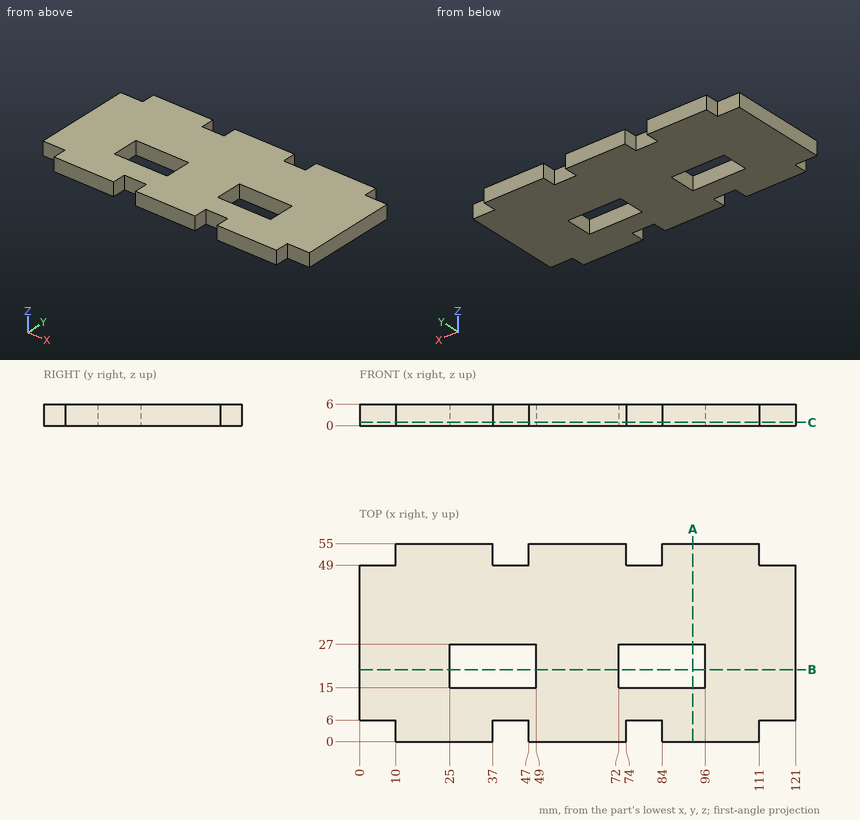
The drawing under review shows one solid part. Ordinate dimensions are in mm from its lowest x, y, z. Round coordinates to 2 decimals unless told otherwise and drop trailing zeros. Write each loop counter-clockwise with the first axis right and the second up, starting at its lowest first coordinate (ties: lowest second). Pieces come first, ordered by that corner, then holes. Notation, with made-up numbers: (-12, -7) - (31, -7) arc R21 cw to (31, 6) - close; hole circle Ø5 at (-23.75, 45.25). An arc over 180 degrees is marked (long way). Use a Markdown table: item, result. Add a question column.
1. We need section A-A (x = 92.5). State the section outline as (y, z) points, then the cut area to 3 significant figures.
2. Wall thickness on probe 1 along X at (y, z) = (53.5, 5.2); probe 2 along X at (y, z) = (24.5, 1.7); probe 3 along Y at (x, z) = (40.5, 2.45): over which ranges is each line inside the solid? List them lowest first.
3. Clearance check with flat-ended pins moving along their axes: pin 1 (1.8 mm diameter, centred on y = 51.5, z = 2, fed in from +X); pin 2 (3 mm diameter, centred on y = 3, z = 4, fed in from -X); pin 3 (3 mm diameter, centred on x = 79, z = 3.5, fed in from -Y). State where each tip first meets the part, or that it passes through.
4. We need section C-C (z = 0.9). Count the separate pieces of the cut face and the enclosed holes in it, then the cut area to 3 significant figures.
5. We need section B-B (y = 20). State the section outline as (x, z) points.
Output:
| question | item | result |
|---|---|---|
| 1 | outline | (0, 0) - (15, 0) - (15, 6) - (0, 6) - close; (27, 0) - (55, 0) - (55, 6) - (27, 6) - close |
| 1 | area | 258 mm2 |
| 2 | probe 1 | x = 10 to 37, 47 to 74, 84 to 111 |
| 2 | probe 2 | x = 0 to 25, 49 to 72, 96 to 121 |
| 2 | probe 3 | y = 6 to 15, 27 to 49 |
| 3 | pin 1 | stops at x = 111 |
| 3 | pin 2 | stops at x = 10 |
| 3 | pin 3 | stops at y = 6 |
| 4 | separate pieces | 1 |
| 4 | enclosed holes | 2 |
| 4 | area | 5,600 mm2 |
| 5 | outline | (0, 0) - (25, 0) - (25, 6) - (0, 6) - close; (49, 0) - (72, 0) - (72, 6) - (49, 6) - close; (96, 0) - (121, 0) - (121, 6) - (96, 6) - close |
